Input: part model. Units: mm. Frame: model coordinates. A direction names the side the tool comes from. Coordinates: 2 decimals unless noted, no trailing zeros. Write each loop counter-clockwise with the first axis right and the second up, starting at its lowest first coordinate (ties: lowest second). Pieces come first, ordered by that corner, then holes. Notation, with made-up numbers: M 85.25,57.5 L 141.25,57.5 A27 ccw 141.25,94.5 Z; hole C 23.5,-26.75 d1. An arc over 180 degrees is marked long. Answer as a JSON object with one key per item and string values. Group by question number.
Autodesk Inventor part; units mm, degrees
ref_plane "YZ Plane" through (0, 0, 0) normal (1, 0, 0) x (0, 1, 0)
ref_plane "XZ Plane" through (0, 0, 0) normal (0, 1, 0) x (-1, 0, 0)
ref_plane "XY Plane" through (0, 0, 0) normal (0, 0, 1) x (1, 0, 0)
ref_plane "Work Plane1" through (-30, 0, 0) normal (0, 0, 1) x (1, 0, 0)
sketch "Sketch1" plane through (-30, 0, 0) normal (0, 0, 1) x (1, 0, 0)
  line L0 (0, 6) -> (10, 6)
  line L1 (0, 0) -> (0, 6)
  line L2 (10, 0) -> (0, 0)
  line L3 (10, 0) -> (10, 6)
  line L4 (30, 6) -> (40, 6)
  line L5 (30, 0) -> (30, 6)
  line L6 (40, 0) -> (30, 0)
  line L7 (40, 0) -> (40, 6)
  line L8 (49, 0) -> (49, -9)
  line L9 (-9, -9) -> (-9, 0)
  line L10 (-15, 0) -> (0, 0)
  line L11 (10, 0) -> (30, 0)
  line L12 (40, 0) -> (55, 0)
  line L13 (121.5157, 6) -> (-97.4843, 6)
  line L14 (-97.4843, -9) -> (121.5157, -9)
  line L15 (25, -9) -> (15, -9)
  line L16 (15, -9) -> (15, -15)
  line L17 (15, -15) -> (25, -15)
  line L18 (25, -15) -> (25, -9)
  point P0 (20, -15)
  point P1 (20, 0)
  dimension "d0" = 10
  dimension "d1" = 6
extrude "Plate1" add sketch "Sketch1" along normal blind 6 contours L0 L3 L2 L1 | L2 L11 L6 L12 L8 L14 L9 L10 | L4 L7 L6 L5 | L14 L18 L17 L16
equation "\"d2\" = Thickness"
equation "\"BendRadius\" = Thickness"
equation "\"BendReliefWidth\" = Thickness"
equation "\"BendReliefDepth\" = 0.5 * Thickness"
equation "\"CornerReliefSize\" = 4 * Thickness"
equation "\"MinimumRemnant\" = 2 * Thickness"
equation "\"TransitionRadius\" = BendRadius"
equation "\"JacobiRadiusSize\" = BendRadius"
equation "\"GapSize\" = Thickness"
properties part number "joystick buiskant" material "Wood (Birch)"
Q1. Section C-C, the plane x = -7.5. Return the cut outline in (y, z), and give its area (3 significant figures).
Q2. Access query for faces 4 (the flat face through (10, 3, 3)), 5 (the flat face through (-5, -12, 3)), 6 (the flat face through (-35, 0, 3)). Directions: +Z, -Z, +X, -X, +Y, -Y. A direction counts if a zero-diameter tool reaches every point of the face in a straight line with its end or side. Return the directions, or none.
Q3. Pin query (flat end, axial travel): pin 1 Ø1.8 at (y, z) = (-13, 4) entering from -X; pin 2 Ø12 at (x, y) = (-22, -9.5) entering from -Z; pin 3 Ø1.8 at (y, z) = (3.5, 3.5) entering from +X; pin 4 Ø1.8 at (x, z) = (-26.5, 3.5) entering from -Y. Return the tip coordinate at first contact, or that it passes through.
Q4. Line query: line 1 (X direction, y = 3.5, z = 2.1); line 2 (Y direction, x = -4.5, z = 5.45); line 3 (Y direction, x = -8.5, z = 5.05). Output: solid intervals per line, ascending. Write a range as from..to.
Q5. Section B-B, the plane z = 4.2. Return the cut outline in (x, y).
Q6. Section A-A, the plane y = 2.75. Return the cut outline in (x, z).
Q7. Draft query along X for faces 1 (the flat face through (-20, 3, 3)), 2 (the flat face through (14, 0, 3)), 3 (the flat face through (-30, 3, 3)). Return one class per face: released by +X, released by -X, zero draft, split by the parting line, or undercut.
Filled in:
{
 "1": {"outline": "M -15,0 L 0,0 L 0,6 L -15,6 Z", "area": "90.0 mm^2"},
 "2": {"face 4": "+Z, -Z, +X, +Y", "face 5": "+Z, -Z, +X, -Y", "face 6": "+Z, -Z, -X, +Y"},
 "3": {"pin 1": "x = -15", "pin 2": "z = 0", "pin 3": "x = 10", "pin 4": "y = -9"},
 "4": {"line 1": "-30..-20, 0..10", "line 2": "-9..0", "line 3": "-15..0"},
 "5": {"outline": "M -39,-9 L -15,-9 L -15,-15 L -5,-15 L -5,-9 L 19,-9 L 19,0 L 10,0 L 10,6 L 0,6 L 0,0 L -20,0 L -20,6 L -30,6 L -30,0 L -39,0 Z"},
 "6": {"outline": "M -30,0 L -20,0 L -20,6 L -30,6 Z; M 0,0 L 10,0 L 10,6 L 0,6 Z"},
 "7": {"face 1": "undercut", "face 2": "zero draft", "face 3": "released by -X"}
}
